Can you work these out from the model? Positions are in its coordinate system, mm. Face numbers are marked on the shaded views. A direction names the side the tool comes from. Coordinates: 2 decimals unless noted, no trailing zeros. Loops run counter-clockwise (first coordinate to the right, second up) from the corner with the lowest first, then second, coordinate; pieces in that order, holes last. Notation, with made-up numbers: M 38.5,85 L 79.5,85 A17 cw 79.5,109 Z; hole C -3.75,16.5 d7. An arc over 180 degrees is marked long. Answer as a JSON object with one key per item and string values. Group by question number.
Item 1: We'd pull the mould along X, two halves only. Please class the marked faces 1, 2 and 3: +X half, -X half, draft (parallel to the pull), parting line (faces both ways), or undercut.
Item 2: Suppose I cut it at B-B (z = -8). Write out the boundary of the cut face in (x, y), then the cut area to 3 significant figures.
Item 3: I'm going to push flat-ended pins straight in: pin 1 Ø3 at (y, z) = (1, -3) entering from -X; pin 2 Ø2.5 at (x, z) = (-4.95, 4.95) entering from -Y. Where does each tip first touch, or does it pass through?
Item 4: Suppose I cut it at D-D (z = 0.5). Write out the boundary of the cut face in (x, y).
Item 5: Which directions (+Z, -Z, +X, -X, +Y, -Y) give clear straight access to the entire face, cutting with the end or side of a thin tool? Please do the marked faces 4 and 5.
Item 6: If I drill on line 1 (X direction, y = 3.7, z = 0); line 2 (Y direction, x = -7.5, z = 2.5), over which ranges is the centre line in solid material (lowest first)?
Item 7: Suppose I cut it at C-C (y = 4.75). Count the separate pieces of the cut face and the enclosed holes in it, then the cut area to 3 significant figures.
Item 8: Suppose I cut it at A-A (x = 0). Write out the boundary of the cut face in (y, z), then the cut area to 3 significant figures.
```python
from build123d import *

# Parameters (mm, degrees)
M2_TAPPED_HOLE1_AT_2_COUNT = 2
M2_TAPPED_HOLE1_AT_2_PITCH = 5.814124225
CIRPATTERN1_COUNT          = 4


with BuildPart() as part:
    # Sketch1 → Revolve1 (revolve)
    with BuildSketch(Plane.XY):
        Polygon((-5, 0), (-5, 3), (-10.5, 3), (-10.5, 5), (0, 5), (0, 0), align=None)
    revolve(axis=Axis((0, 5, 0), (0, -1, 0)))

    # Sketch4 → M2 Tapped Hole1 (revolve, cut)
    with BuildSketch(Plane(origin=(8, 5, 0), x_dir=(0, 0, 1), z_dir=(1, 0, 0))):
        Polygon((0, 0), (0, 6.480688495), (0.8, 6), (0.8, 0), align=None)
    m2_tapped_hole1 = revolve(axis=Axis((8, 11.35, 0), (0, -1, 0)), mode=Mode.SUBTRACT)

    # M2 Tapped Hole1 at 2: M2 Tapped Hole1 ×2
    with Locations(*[Vector(-0.524628029, 0, 0.851331564) * (i * M2_TAPPED_HOLE1_AT_2_PITCH) for i in range(1, M2_TAPPED_HOLE1_AT_2_COUNT)]):
        add(m2_tapped_hole1, mode=Mode.SUBTRACT)

    # CirPattern1: M2 Tapped Hole1 ×4 about axis
    cirpattern1_axis = Axis((0, 0, 0), (0, 1, 0))
    for i in range(1, CIRPATTERN1_COUNT):
        add(m2_tapped_hole1.rotate(cirpattern1_axis, i * 360 / CIRPATTERN1_COUNT), mode=Mode.SUBTRACT)

    # CirPattern1 copy 1 sketch → CirPattern1 copy 1 (revolve, cut)
    with BuildSketch(Plane(origin=(4.949747468, 5, -4.949747468), x_dir=(1, 0, 0), z_dir=(0, 0, -1))):
        Polygon((0, 0), (0, 6.480688495), (0.8, 6), (0.8, 0), align=None)
    revolve(axis=Axis((4.949747468, 11.35, -4.949747468), (0, -1, 0)), mode=Mode.SUBTRACT)

    # CirPattern1 copy 2 sketch → CirPattern1 copy 2 (revolve, cut)
    with BuildSketch(Plane(origin=(-4.949747468, 5, -4.949747468), x_dir=(0, 0, -1), z_dir=(-1, 0, 0))):
        Polygon((0, 0), (0, 6.480688495), (0.8, 6), (0.8, 0), align=None)
    revolve(axis=Axis((-4.949747468, 11.35, -4.949747468), (0, -1, 0)), mode=Mode.SUBTRACT)

    # CirPattern1 copy 3 sketch → CirPattern1 copy 3 (revolve, cut)
    with BuildSketch(Plane(origin=(-4.949747468, 5, 4.949747468), x_dir=(-1, 0, 0), z_dir=(0, 0, 1))):
        Polygon((0, 0), (0, 6.480688495), (0.8, 6), (0.8, 0), align=None)
    revolve(axis=Axis((-4.949747468, 11.35, 4.949747468), (0, -1, 0)), mode=Mode.SUBTRACT)


solid = part.part
```
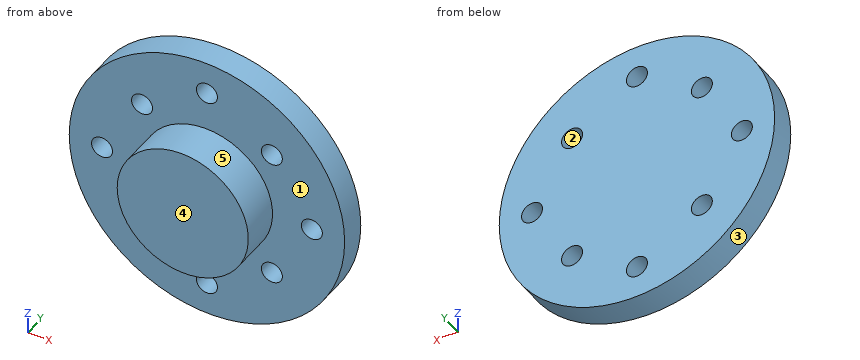
From the geometry:
{
 "1": {"face 1": "draft", "face 2": "undercut", "face 3": "parting line"},
 "2": {"outline": "M -6.8,3 L -0.8,3 L -0.8,5 L -6.8,5 Z; M 0.8,3 L 6.8,3 L 6.8,5 L 0.8,5 Z", "area": "24.0 mm2"},
 "3": {"pin 1": "x = -4.77", "pin 2": "y = 3"},
 "4": {"outline": "M -10.49,3 L -8.62,3 L -8.62,5 L -10.49,5 Z; M -7.38,3 L -4.97,3 L -4.97,0 L 4.97,0 L 4.97,3 L 7.38,3 L 7.38,5 L -7.38,5 Z; M 8.62,3 L 10.49,3 L 10.49,5 L 8.62,5 Z"},
 "5": {"face 4": "+Z, -Z, +X, -X, -Y", "face 5": "-Y"},
 "6": {"line 1": "-10.5 to -8.8, -7.2 to 7.2, 8.8 to 10.5", "line 2": "3 to 5"},
 "7": {"separate pieces": "1", "enclosed holes": "8", "area": "330 mm2"},
 "8": {"outline": "M 0,-5 L 3,-5 L 3,-7.2 L 5,-7.2 L 5,7.2 L 3,7.2 L 3,5 L 0,5 Z; M 3,-10.5 L 5,-10.5 L 5,-8.8 L 3,-8.8 Z; M 3,8.8 L 5,8.8 L 5,10.5 L 3,10.5 Z", "area": "65.6 mm2"}
}
